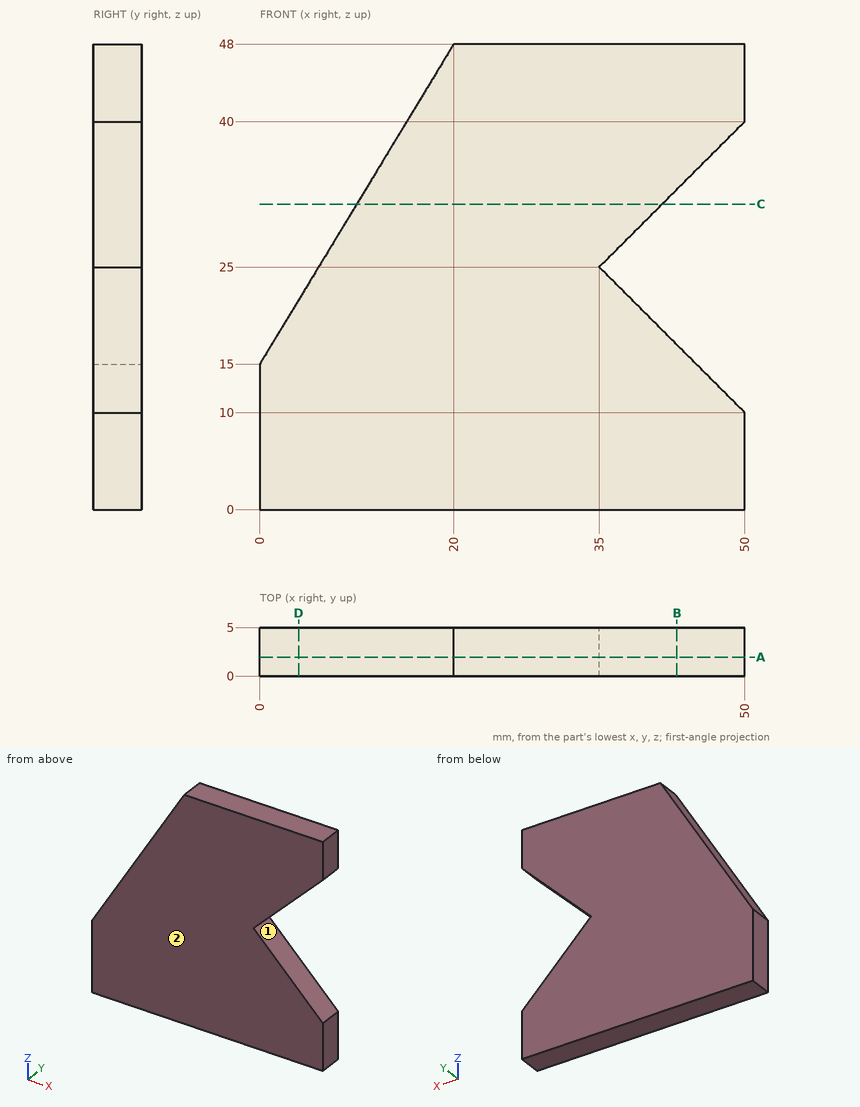
Verification items for this drawing (mm, ordinates from the low corner). A direction names the side the tool comes from. Round coordinates to 2 decimals unless told otherwise and drop trailing zeros. Loops run counter-clockwise (first coordinate to the right, second up) from the corner with the lowest first, then second, coordinate; pieces in that order, holes last. Notation, with made-up numbers: (84, 24.25) -> (97, 24.25) arc R20 ccw to (97, 58.25) -> close; hole circle Ø3 at (-9, 33.25). An arc over 180 degrees is marked (long way). Write item = value, one per line. Start each with the question number.
1) Set-up check for the marked faces 1 and 2: record each of +Z, -Z, +X, -X, +Y, -Y from which the full face is reachable in a straight line by a thin tool's end or side.
2) Gauge pin test, flat ends, axial feed: pin 1 Ø4 at (x, z) = (36.5, 7) entering from -Y; pin 2 Ø1 at (y, z) = (2.5, 33) entering from -X; pin 3 Ø1.5 at (y, z) = (2, 22.5) entering from -X. Record the tip position at first contact, or that the pin passes through.
3) Sectioned sample at A-A, the plane y = 1.95. Record the cut outline in (x, z), plus the area to 4 significant figures.
4) Sectioned sample at B-B, the plane x = 43. Record the cut outline in (y, z).
5) Sectioned sample at C-C, the plane z = 31.5. Record the cut outline in (x, y).
6) Sectioned sample at D-D, the plane x = 4. Record the cut outline in (y, z), plus the area to 3 significant figures.
7) Thickness scan on probe 1 along X at (y, z) = (0.7, 12); probe 2 along Z at (x, y) = (36, 1.15); probe 3 along X at (y, z) = (1.5, 29.5). Record the ranges inside material, lowest first.
Results are:
q1.face_1 = +X, +Y, -Y
q1.face_2 = +Z, -Z, +X, -X, -Y
q2.pin_1 = 0
q2.pin_2 = 10.61
q2.pin_3 = 4.09
q3.outline = (0, 0) -> (50, 0) -> (50, 10) -> (35, 25) -> (50, 40) -> (50, 48) -> (20, 48) -> (0, 15) -> close
q3.area = 1,845 mm^2
q4.outline = (0, 0) -> (5, 0) -> (5, 17) -> (0, 17) -> close; (0, 33) -> (5, 33) -> (5, 48) -> (0, 48) -> close
q5.outline = (10, 0) -> (41.5, 0) -> (41.5, 5) -> (10, 5) -> close
q6.outline = (0, 0) -> (5, 0) -> (5, 21.6) -> (0, 21.6) -> close
q6.area = 108 mm^2
q7.probe_1 = 0 to 48
q7.probe_2 = 0 to 24, 26 to 48
q7.probe_3 = 8.79 to 39.5
